Geometry check sheet. Reference: the model listing, model coordinates, mm. Give positions to 0.01 mm unless a question says otherwise; leave off trailing zeros. Loops run counter-clockwise (first coordinate to the right, second up) from the corner with the lowest first, then second, coordinate; pieces in that order, holes last. Notation, with made-up numbers: (-8.75, 13.5) -> (37.25, 13.5) arc R13 ccw to (37.25, 35.5) -> close; hole circle Ø4 at (-10.75, 74.5). An arc over 180 degrees is marked (long way). Write item = value, one per line.
```python
from build123d import *

# Parameters (mm, degrees)
SKETCH_2_R      = 1.5
SKETCH_2_R_2    = 20
SKETCH_2_R_3    = 2.3
EXTRUDE_1_DEPTH = 3


with BuildPart() as part:
    # 草图2 → 凸台-拉伸1 (new body)
    with BuildSketch(Plane(origin=(0, 0, 0), x_dir=(1, 0, 0), z_dir=(0, 1, 0))):
        with BuildLine():
            ThreePointArc((60.260378076, 43.805671256), (0, 74.5), (-60.260378076, 43.805671256))
            ThreePointArc((-60.260378076, 43.805671256), (-48.360726818, 0), (-60.260378076, -43.805671256))
            ThreePointArc((-60.260378076, -43.805671256), (0, -74.5), (60.260378076, -43.805671256))
            ThreePointArc((60.260378076, -43.805671256), (48.360726818, 0), (60.260378076, 43.805671256))
        make_face()
        with Locations(Location((0, 71.5, 0), (0, 0, 270))):
            Circle(SKETCH_2_R, mode=Mode.SUBTRACT)
        with Locations(Location((50.558134855, 50.558134855, 0), (0, 0, 270))):
            Circle(SKETCH_2_R, mode=Mode.SUBTRACT)
        with Locations(Location((50.558134855, -50.558134855, 0), (0, 0, 270))):
            Circle(SKETCH_2_R, mode=Mode.SUBTRACT)
        with Locations(Location((0, -71.5, 0), (0, 0, 270))):
            Circle(SKETCH_2_R, mode=Mode.SUBTRACT)
        with Locations(Location((-50.558134855, -50.558134855, 0), (0, 0, 270))):
            Circle(SKETCH_2_R, mode=Mode.SUBTRACT)
        with Locations(Location((-50.558134855, 50.558134855, 0), (0, 0, 270))):
            Circle(SKETCH_2_R, mode=Mode.SUBTRACT)
        with Locations(Location((0, 0, 0), (0, 0, 270))):
            Circle(SKETCH_2_R_2, mode=Mode.SUBTRACT)
        with Locations(Location((-23.55, 23.55, 0), (0, 0, 270))):
            Circle(SKETCH_2_R_3, mode=Mode.SUBTRACT)
        with Locations(Location((23.55, 23.55, 0), (0, 0, 270))):
            Circle(SKETCH_2_R_3, mode=Mode.SUBTRACT)
        with Locations(Location((23.55, -23.55, 0), (0, 0, 270))):
            Circle(SKETCH_2_R_3, mode=Mode.SUBTRACT)
        with Locations(Location((-23.55, -23.55, 0), (0, 0, 270))):
            Circle(SKETCH_2_R_3, mode=Mode.SUBTRACT)
    extrude(amount=EXTRUDE_1_DEPTH)


solid = part.part
```
Item 1: Section check A-A, the plane z = 0. Record the cut outline in (x, y).
Answer:
outline = (-48.36, 0) -> (-20, 0) -> (-20, 3) -> (-48.36, 3) -> close; (20, 0) -> (48.36, 0) -> (48.36, 3) -> (20, 3) -> close
Item 2: Section check D-D, the plane z = -23.55. Record the cut outline in (x, y), plus the area to 3 significant figures.
Answer:
outline = (-51.63, 0) -> (-25.85, 0) -> (-25.85, 3) -> (-51.63, 3) -> close; (-21.25, 0) -> (21.25, 0) -> (21.25, 3) -> (-21.25, 3) -> close; (25.85, 0) -> (51.63, 0) -> (51.63, 3) -> (25.85, 3) -> close
area = 282 mm^2
Item 3: Section check B-B, the plane x = -23.55. Record the cut outline in (y, z).
Answer:
outline = (0, -70.68) -> (3, -70.68) -> (3, -25.85) -> (0, -25.85) -> close; (0, -21.25) -> (3, -21.25) -> (3, 21.25) -> (0, 21.25) -> close; (0, 25.85) -> (3, 25.85) -> (3, 70.68) -> (0, 70.68) -> close
Item 4: Section check C-C, the plane y = 0.95. Give the number of separate pieces and of enclosed holes in the cut face, plus the area to 3 significant figures.
Answer:
separate_pieces = 1
enclosed_holes = 11
area = 13,000 mm^2
Item 5: Draft check along X on faces 1 (the cylindrical face through (-50.49, 1.48, 49.06)), 2 (the cylindrical face through (-48.363, 1.479, -0.643)), 3 (the flat face through (-14, 0, -18)). Enter one of: +X half, -X half, draft (parallel to the pull), parting line (faces both ways), or undercut.
Answer:
face_1 = undercut
face_2 = -X half
face_3 = draft
Item 6: Gauge pin test, flat ends, axial feed: pin 1 (3 mm diameter, centred on x = 23.55, z = -23.55, fed in from +Y); pin 2 (4 mm diameter, centred on x = -50.56, z = 50.56, fed in from +Y). Record the tip position at first contact, or that the pin passes through.
Answer:
pin_1 = through
pin_2 = 3
Item 7: Thickness scan on L1, parallel to X at y = 0.75, z = 23.55; L2, parallel to X at y = 2.05, z = -21.5; L3, parallel to X at y = 2.95, z = -13. Record the ranges inside material, lowest first. Write a range as [from, to].
Answer:
L1 = [-51.63, -25.85], [-21.25, 21.25], [25.85, 51.63]
L2 = [-51.07, -24.59], [-22.51, 22.51], [24.59, 51.07]
L3 = [-49.34, -15.2], [15.2, 49.34]
